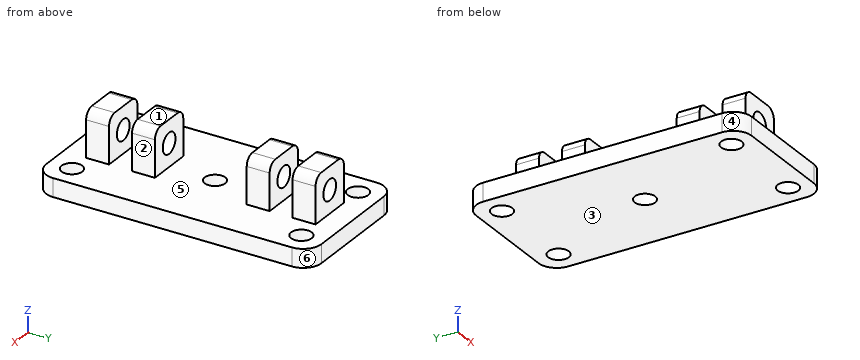
```python
from build123d import *

# Parameters (mm, degrees)
ESQUISSE1_W             = 30
ESQUISSE1_H             = 60
BOSS_EXTRU_1_DEPTH      = 4
ESQUISSE2_W             = 10
ESQUISSE2_H             = 5
BOSS_EXTRU_2_DEPTH      = 10
ESQUISSE3_R             = 2.25
ENL_V_MAT_EXTRU_1_DEPTH = 56
CONG_1_R                = 2
CONG_2_R                = 4
ESQUISSE4_R             = 2.25
ENL_V_MAT_EXTRU_2_DEPTH = 5


with BuildPart() as part:
    # Esquisse1 → Boss.-Extru.1 (new body)
    with BuildSketch(Plane.XY):
        with Locations((-15, 30)):
            Rectangle(ESQUISSE1_W, ESQUISSE1_H)
    extrude(amount=BOSS_EXTRU_1_DEPTH)

    # Esquisse2 → Boss.-Extru.2 (add)
    with BuildSketch(Plane.XY.offset(4)):
        with Locations((-15, 52.5)):
            Rectangle(ESQUISSE2_W, ESQUISSE2_H)
        with Locations((-15, 42.5)):
            Rectangle(ESQUISSE2_W, ESQUISSE2_H)
        with Locations((-15, 17.5)):
            Rectangle(ESQUISSE2_W, ESQUISSE2_H)
        with Locations((-15, 7.5)):
            Rectangle(ESQUISSE2_W, ESQUISSE2_H)
    extrude(amount=BOSS_EXTRU_2_DEPTH)

    # Esquisse3 → Enlèv. mat.-Extru.1 (cut, through all)
    with BuildSketch(Plane.XZ.offset(-5)):
        with Locations(Location((-15, 9, 0), (0, 0, 270))):  # turned: the seam where the file's is
            Circle(ESQUISSE3_R)
    extrude(amount=-ENL_V_MAT_EXTRU_1_DEPTH, mode=Mode.SUBTRACT)

    # Congé1
    cong_1_edges = [part.edges().sort_by_distance(p)[0] for p in [
        (-20, 52.5, 14),
        (-10, 52.5, 14),
        (-20, 42.5, 14),
        (-10, 42.5, 14),
        (-20, 17.5, 14),
        (-10, 17.5, 14),
        (-20, 7.5, 14),
        (-10, 7.5, 14),
    ]]
    fillet(cong_1_edges, radius=CONG_1_R)

    # Congé2
    cong_2_edges = [part.edges().sort_by_distance(p)[0] for p in [
        (-30, 60, 2),
        (0, 60, 2),
        (0, 0, 2),
        (-30, 0, 2),
    ]]
    fillet(cong_2_edges, radius=CONG_2_R)

    # Esquisse4 → Enlèv. mat.-Extru.2 (cut, through all)
    with BuildSketch(Plane.XY.offset(4)):
        with Locations((-5, 55)):
            Circle(ESQUISSE4_R)
        with Locations((-25, 55)):
            Circle(ESQUISSE4_R)
        with Locations((-5, 5)):
            Circle(ESQUISSE4_R)
        with Locations((-25, 5)):
            Circle(ESQUISSE4_R)
        with Locations((-15, 30)):
            Circle(ESQUISSE4_R)
    extrude(amount=-ENL_V_MAT_EXTRU_2_DEPTH, mode=Mode.SUBTRACT)


solid = part.part
```
Geometry check sheet. Reference: the model listing, model coordinates, mm. Face numbers are marked on the shaded views. A direction names the side the tool comes from. Round coordinates to 2 decimals unless told otherwise and drop trailing zeros. Order: outer loops, then holes, each group sorted by start corner. A loop starts at its lowest first (then second) coordinate and runs counter-clockwise, first axis right, second up. Notation, with made-up numbers: (-29.5, -38.75) - (-2.5, -38.75) arc R29 ccw to (-2.5, -17.75) - close; hole circle Ø11 at (-35.75, 43). An arc over 180 degrees is marked (long way). Use a Markdown table: item, result. Add a question column.
1) Section check B-B (z = 9). Count the separate pieces of the cut face and the enclosed holes in it, then the cut area to 3 significant figures.
2) Thickness scan on line 1 along Y through (x, z) = (-15.25, 5); line 2 along Y through (x, z) = (-25, 1.9); line 3 along X through (y, z) = (7.4, 9). Record the ranges inside material, lowest first.
3) Set-up check for the marked faces 1 and 2: record each of +Z, -Z, +X, -X, +Y, -Y from which the full face is reachable in a straight line by a thin tool's end or side.
4) Section check A-A (y = 53.5). Record the cut outline in (x, z).
5) Section check C-C (x = -5). Record the cut outline in (y, z).
6) Gauge pin test, flat ends, axial feed: P1, Ø8, axis at x = -15.5, z = 10, coming from the -Y side; P2, Ø12, axis at x = -7.5, y = 23.5, coming from the -Z side; P3, Ø4, axis at y = 17.5, z = 8, coming from the -X side; P4, Ø2.5, axis at x = -25, y = 55, coming from the +Z side. Record the tip position at first contact, or that the pin passes through.
7) Section check D-D (z = 5.5). Record the cut outline in (x, y), then the cut area to 3 significant figures.
8) Mould release check, pull along Y, two halves, no side actions. Record for the marked faces 3, 4, 5 and 6: released by +Y, released by -Y, zero draft, split by the parting line, or undercut.
Established:
| question | item | result |
|---|---|---|
| 1 | separate pieces | 8 |
| 1 | enclosed holes | 0 |
| 1 | area | 110 mm2 |
| 2 | line 1 | 5 to 10, 15 to 20, 40 to 45, 50 to 55 |
| 2 | line 2 | 0 to 2.75, 7.25 to 52.75, 57.25 to 60 |
| 2 | line 3 | -20 to -17.25, -12.75 to -10 |
| 3 | face 1 | +Z, +X, -X, +Y, -Y |
| 3 | face 2 | +Z, +X, +Y, -Y |
| 4 | outline | (-30, 0) - (-26.68, 0) - (-26.68, 4) - (-30, 4) - close; (-23.32, 0) - (-6.68, 0) - (-6.68, 4) - (-10, 4) - (-10, 12) arc R2 ccw to (-12, 14) - (-18, 14) arc R2 ccw to (-20, 12) - (-20, 4) - (-23.32, 4) - close; (-3.32, 0) - (0, 0) - (0, 4) - (-3.32, 4) - close; hole circle Ø4.5 at (-15, 9) |
| 5 | outline | (0, 0) - (2.75, 0) - (2.75, 4) - (0, 4) - close; (7.25, 0) - (52.75, 0) - (52.75, 4) - (7.25, 4) - close; (57.25, 0) - (60, 0) - (60, 4) - (57.25, 4) - close |
| 6 | P1 | y = 5 |
| 6 | P2 | z = 0 |
| 6 | P3 | x = -20 |
| 6 | P4 | through |
| 7 | outline | (-20, 5) - (-10, 5) - (-10, 10) - (-20, 10) - close; (-20, 15) - (-10, 15) - (-10, 20) - (-20, 20) - close; (-20, 40) - (-10, 40) - (-10, 45) - (-20, 45) - close; (-20, 50) - (-10, 50) - (-10, 55) - (-20, 55) - close |
| 7 | area | 200 mm2 |
| 8 | face 3 | zero draft |
| 8 | face 4 | released by -Y |
| 8 | face 5 | undercut |
| 8 | face 6 | released by +Y |
